Read the model definition and answer for the solid it produces. Units are mm, in the model's axes. Round coordinates to 2 decimals unless told otherwise and drop trailing zeros. Loops run counter-clockwise (first coordinate to the right, second up) from the corner with the lowest first, then second, coordinate; pieces in that order, holes last. Notation, with made-up numbers: (89, 40.25) -> (100, 40.25) arc R22 cw to (100, 79.25) -> close; hole circle Ø3 at (76.5, 2). An arc over 180 degrees is marked (long way). Put each result on its own line as item: value.
Autodesk Inventor part; units mm, degrees
ref_plane "YZ Plane" through (0, 0, 0) normal (1, 0, 0) x (0, 1, 0)
ref_plane "XZ Plane" through (0, 0, 0) normal (0, 1, 0) x (-1, 0, 0)
ref_plane "XY Plane" through (0, 0, 0) normal (0, 0, 1) x (1, 0, 0)
sketch "Sketch1" plane through (0, 0, 0) normal (0, 1, 0) x (-1, 0, 0)
  line L0 (1.75, 0) -> (34.25, 0)
  line L1 (36, -1.75) -> (36, -58.25)
  line L2 (34.25, -60) -> (1.75, -60)
  line L3 (0, -58.25) -> (0, -1.75)
  arc A0 (36, -1.75) -> (34.25, 0) centre (34.25, -1.75) ccw
  arc A1 (1.75, 0) -> (0, -1.75) centre (1.75, -1.75) ccw
  arc A2 (0, -58.25) -> (1.75, -60) centre (1.75, -58.25) ccw
  arc A3 (34.25, -60) -> (36, -58.25) centre (34.25, -58.25) ccw
  point P0 (0, 0)
  point P1 (36, -60)
  point P2 (36, 0)
  point P3 (0, -60)
  dimension "d0" = 36
  dimension "d1" = 60
  dimension "d2" = 1.75
extrude "Extrusion1" add sketch "Sketch1" along normal blind 1.6
sketch "Sketch2" plane through (0, 1.6, 0) normal (0, 1, 0) x (1, 0, 0)
  line L0 (-32.5, 3.75) -> (-3.5, 3.75) construction
  line L1 (-3.5, 3.75) -> (-3.5, 56.25) construction
  line L2 (-3.5, 56.25) -> (-32.5, 56.25) construction
  line L3 (-32.5, 56.25) -> (-32.5, 3.75) construction
  line L4 (-36, 58.25) -> (-36, 1.75)
  line L5 (0, 1.75) -> (0, 58.25)
  line L6 (-1.75, 60) -> (-34.25, 60)
  line L7 (-34.25, 0) -> (-1.75, 0)
  point P0 (0, 0)
  dimension "d5" = 52.5
  dimension "d6" = 29
  dimension "d7" = 36
  dimension "d8" = 60
  dimension "d9" = 3.75
  dimension "d10" = 3.5
hole "Hole1" at (-32.5, 1.6, -3.75) at (-3.5, 1.6, -3.75) at (-3.5, 1.6, -56.25) at (-32.5, 1.6, -56.25) direction (0, -1, 0) diameter 2.459 depth 8.8
equation "\"d9\" = -0.5 * d5 + 0.5 * d8"
equation "\"d10\" = -0.5 * d6 + 0.5 * d7"
properties part number "Drok Step Down PCB"
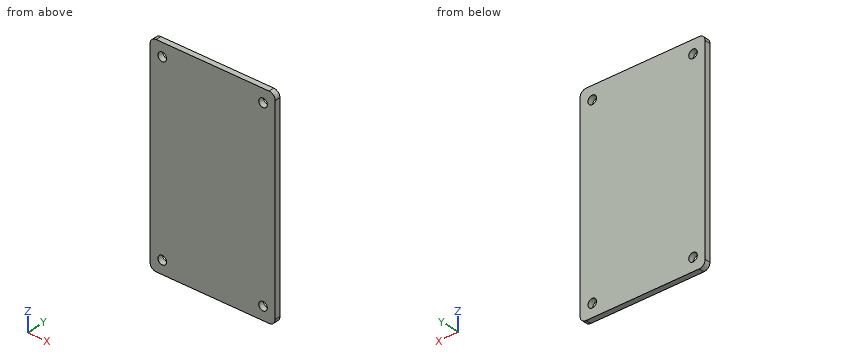
Item 1: The part is cut by section A-A (z = -3.75). Determine the outline of the cut face in (x, y), then the cut area to 3 significant figures.
Derived:
outline: (-36, 0) -> (-33.73, 0) -> (-33.73, 1.6) -> (-36, 1.6) -> close; (-31.27, 0) -> (-4.73, 0) -> (-4.73, 1.6) -> (-31.27, 1.6) -> close; (-2.27, 0) -> (0, 0) -> (0, 1.6) -> (-2.27, 1.6) -> close
area: 49.7 mm^2
Item 2: Find the intervals of material crossed by line 1 along Z through (x, y) = (-3.5, 0.4); line 2 along X through (y, z) = (0.4, -56.25); line 3 along Z through (x, y) = (-4, 1.15), in increasing order.
Derived:
line 1: z = -60 to -57.48, -55.02 to -4.98, -2.52 to 0
line 2: x = -36 to -33.73, -31.27 to -4.73, -2.27 to 0
line 3: z = -60 to -57.37, -55.13 to -4.87, -2.63 to 0
Item 3: A flat-ended cylindrical pin translates along its axis: pin 1 Ø3 at (x, z) = (-13, -21) entering from -Y. Find the tip coordinate at first contact, or state that the pin passes through.
Derived:
pin 1: stops at y = 0
Item 4: The part is cut by section B-B (x = -3.5). Determine the outline of the cut face in (y, z).
Derived:
outline: (0, -60) -> (1.6, -60) -> (1.6, -57.48) -> (0, -57.48) -> close; (0, -55.02) -> (1.6, -55.02) -> (1.6, -4.98) -> (0, -4.98) -> close; (0, -2.52) -> (1.6, -2.52) -> (1.6, 0) -> (0, 0) -> close
